Input: part model. Units: mm. Frame: model coordinates. A direction names the side the tool comes from. Give positions to 0.01 mm unless a question says otherwise; leave off trailing zeros. Order: outer loops, then holes, each group sorted by start corner. A loop starts at its lowest first (then second) coordinate and runs counter-clockwise, first axis right, second up. Notation, with made-up numbers: (63, 12.25) - (78, 12.25) arc R20 ccw to (78, 34.25) - close; hole circle Ø9 at (-37.5, 48). An arc over 180 degrees is marked (long way). Use a Markdown table: item, result.
from build123d import *

# Parameters (mm, degrees)
F3_D     = 8.5
F4_SIZE2 = 0.5358983849
F4_SIZE  = 2


with BuildPart() as f1:
    # F0 (on Front) → F1 (revolve)
    with BuildSketch(Plane.XZ):
        Polygon((0, 17), (0, 0), (16, 0), (16, 15.975), (3, 15.975), (3, 17), align=None)
    revolve(axis=Axis((8, 0, 0), (1, 0, 0)))

    # F3 (through all)
    with Locations(Plane.YZ.offset(16)):
        with Locations((0, 0)):
            Hole(F3_D / 2)

    # F4
    f4_edges = [f1.edges().sort_by_distance(p)[0] for p in [
        (16, 0, -15.975),
    ]]
    f4_side = f1.faces().sort_by_distance((9.5, 0, -15.975))[0]
    chamfer(f4_edges, length=F4_SIZE, length2=F4_SIZE2, reference=f4_side)


solid = f1.part
1. Section query D-D (x = 6.75). Return loops of the section in (y, z) (3 decimals), then the cut area to 3 significant figures.
Response:
| item | result |
|---|---|
| outline | circle Ø31.95 at (0, 0); hole circle Ø8.5 at (0, 0) |
| area | 745 mm^2 |
2. Section query C-C (x = 2). Return loops of the section in (y, z).
Response:
| item | result |
|---|---|
| outline | circle Ø34 at (0, 0); hole circle Ø8.5 at (0, 0) |
3. Section query A-A (z = 0). Return loops of the section in (x, y) (3 decimals), then the cut area to 3 significant figures.
Response:
| item | result |
|---|---|
| outline | (0, -17) - (3, -17) - (3, -15.975) - (14, -15.975) - (16, -15.439) - (16, -4.25) - (0, -4.25) - close; (0, 4.25) - (16, 4.25) - (16, 15.439) - (14, 15.975) - (3, 15.975) - (3, 17) - (0, 17) - close |
| area | 380 mm^2 |
4. Mould query, pull axis Y, two halves, no side actions, for faces 3 (the face through (7.888, -2.285, 3.584)), 4 (the face through (1.479, -14.334, 9.139)), 5 (the face through (16, 3.2, -3.2)). Classes: pulls with the +Y half, pulls with the -Y half, needs draft (parallel to the pull), parting line crosses it, or undercut.
Response:
| item | result |
|---|---|
| face 3 | undercut |
| face 4 | parting line crosses it |
| face 5 | needs draft |
5. Set-up query: faces 1 (the face through (0, 4, 4)), 2 (the face through (8.423, 15.595, -3.463)). Return all of +Z, -Z, +X, -X, +Y, -Y with unobstructed straight access to the full face (end or side cutting, diameter ignored); none if empty.
Response:
| item | result |
|---|---|
| face 1 | +Z, -Z, -X, +Y, -Y |
| face 2 | +X |
6. Material intervals for line 1 along Z through (x, y) = (3.75, 0) (3 decimals); line 2 along Y through (x, z) = (13.25, 0.5); line 3 along Y through (x, z) = (3.75, 1), sorted ascending.
Response:
| item | result |
|---|---|
| line 1 | z = -15.975 to -4.25, 4.25 to 15.975 |
| line 2 | y = -15.97 to -4.22, 4.22 to 15.97 |
| line 3 | y = -15.94 to -4.13, 4.13 to 15.94 |
7. Pin query (flat end, axial travel): pin 1 (10 mm diameter, centred on y = -0.5, z = 1.5, fed in from +X); pin 2 (5 mm diameter, centred on x = 14, z = 8.5, fed in from -Y); pin 3 (6 mm diameter, centred on x = 13, y = -12, fed in from +Z); pin 4 (1.5 mm diameter, centred on x = 8.5, y = 13, fed in from -Z). Return the tip coordinate at first contact, or that it passes through.
Response:
| item | result |
|---|---|
| pin 1 | stops at x = 16 |
| pin 2 | stops at y = -14.81 |
| pin 3 | stops at z = 13.2 |
| pin 4 | stops at z = -10.25 |
